from build123d import *

# Parameters (mm, degrees)
BOX112015002006_W          = 23
BOX112015002006_H          = 34
BOX112015002006_DEPTH      = 80
BOX112015002006_ROLL_ANGLE = -29
BOX112015002005_W          = 21
BOX112015002005_H          = 34
BOX112015002005_DEPTH      = 80
FILLET002_R                = 4


with BuildPart() as cube076:
    # Box112015002006 → Box112015002006 (new body)
    with BuildSketch(Plane.XY):
        with Locations((11.5, 17)):
            Rectangle(BOX112015002006_W, BOX112015002006_H)
    extrude(amount=BOX112015002006_DEPTH)


with BuildPart() as cube076_1:
    # Box112015002006 roll: moved
    add(cube076.part.rotate(Axis((0, 0, 0), (1, 0, 0)), BOX112015002006_ROLL_ANGLE))


with BuildPart() as cube076_2:
    # Box112015002006 placement: moved
    add(cube076_1.part.moved(Location((10, -48, -6))))


with BuildPart() as fillet002:
    # Box112015002005 → Box112015002005 (new body)
    with BuildSketch(Plane(origin=(11, -17, -38), x_dir=(1, 0, 0), z_dir=(0, 0, 1))):
        with Locations((10.5, 17)):
            Rectangle(BOX112015002005_W, BOX112015002005_H)
    extrude(amount=BOX112015002005_DEPTH)

    # Cut131: cut Cube076
    add(cube076_2.part, mode=Mode.SUBTRACT)

    # Fillet002
    fillet002_edges = [fillet002.edges().sort_by_distance(p)[0] for p in [
        (21.5, 17, 41.132483),
    ]]
    fillet(fillet002_edges, radius=FILLET002_R)


with BuildPart() as fillet002_1:
    # Fillet002 placement: moved
    add(fillet002.part.moved(Location((0, 0, 10))))


solid = fillet002_1.part
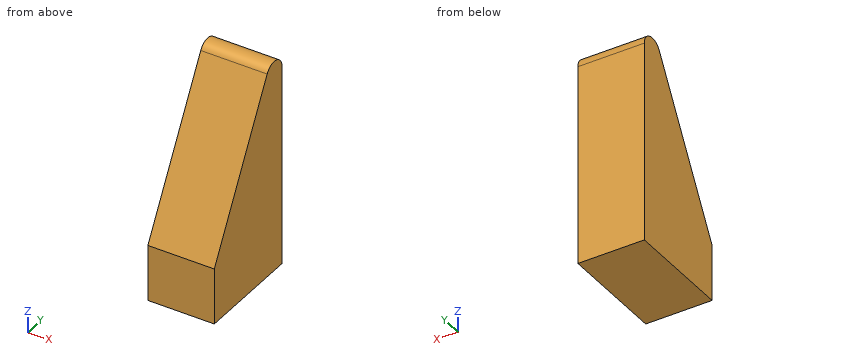
CAD build for the part. Positions are in the model's coordinates, mm. Give positions to 0.01 mm unless a question says otherwise; leave off trailing zeros. Loops run counter-clockwise (first coordinate to the right, second up) from the corner with the lowest first, then second, coordinate; pieces in that order, holes last. Notation, with made-up numbers: M 12,32 L 40,32 A7 ccw 40,44 Z; hole C 61.25,62.25 d4. An arc over 180 degrees is marked long. One line per question, with ' | ' between items. Start each with the question number.
1. Flat gauge pins, fed straight in: pin 1 (3 mm diameter, centred on x = 19, z = 0.5, fed in from -Y); pin 2 (3 mm diameter, centred on x = 23.5, y = 10.5, fed in from +Z); pin 3 (10 mm diameter, centred on x = 16.5, y = -2.5, fed in from +Z). Where does each tip first touch, or does it go through?
2. Saw through at B-B on y = -13.5. Give the cut face in (x, z).
3. Saw through at A-A on x = 19.5. Give the cut face in (y, z), plus the area to 3 significant figures.
4. Probe L1, parallel to Z at x = 19.25, y = 16.5; L2, parallel to Z at x = 21, y = 4; L3, parallel to Y at x = 26.25, z = 21.5. List the from-to ranges inside material, lowest first. Write a range as from..to.
5. Saw through at C-C on z = 11. Give the cut face in (x, y).
Result sheet:
1) pin 1: stops at y = -11.9 | pin 2: stops at z = 39.54 | pin 3: stops at z = 24.97
2) outline: M 11,-28 L 32,-28 L 32,-3.89 L 11,-3.89 Z
3) outline: M -17,-28 L 17,-28 L 17,35.67 A4 ccw 9.5,37.6 L -17,-10.21 Z | area: 1,610 mm^2
4) L1: z = -28..37.6 | L2: z = -28..27.68 | L3: y = 0.57..17
5) outline: M 11,-5.25 L 32,-5.25 L 32,17 L 11,17 Z
